from build123d import *

# Parameters (mm, degrees)
F0_W     = 23.8125
F0_H     = 7.9375
F0_R     = 2.38125
F1_DEPTH = 3.175
F2_DEPTH = 4.7625
F3_T     = -1.5875


with BuildPart() as f1:
    # F0 (on Top) → F1 (new body)
    with BuildSketch(Plane.XY):
        Rectangle(F0_W, F0_H)
        with Locations((-7.9375, 0)):
            Circle(F0_R, mode=Mode.SUBTRACT)
        Circle(F0_R, mode=Mode.SUBTRACT)
        with Locations((7.9375, 0)):
            Circle(F0_R, mode=Mode.SUBTRACT)
    extrude(amount=F1_DEPTH)

    # F0 (on Top) → F2 (join)
    with BuildSketch(Plane.XY):
        with Locations((-7.9375, 0)):
            Circle(F0_R)
        Circle(F0_R)
        with Locations((7.9375, 0)):
            Circle(F0_R)
    extrude(amount=F2_DEPTH)

    # F3
    f3_openings = [f1.faces().sort_by_distance(p)[0] for p in [
        (0, 0, 0),
    ]]
    offset(amount=F3_T, openings=f3_openings, kind=Kind.INTERSECTION)


solid = f1.part
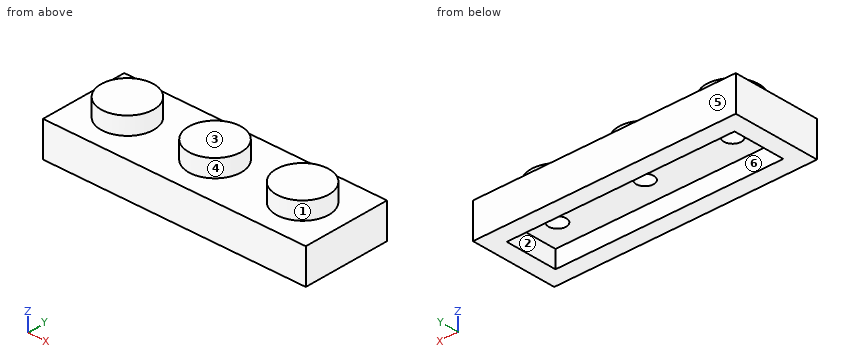
Design review of the part built by this model. Coordinates are the model's own, in mm. Face numbers are marked on the shaded views. A direction names the side the tool comes from. Give positions to 0.01 mm unless a question says otherwise; leave off trailing zeros. Loops run counter-clockwise (first coordinate to the right, second up) from the corner with the lowest first, then second, coordinate; pieces in that order, holes last. Notation, with made-up numbers: (-37.5, 53) -> (1.5, 53) arc R10 cw to (1.5, 65) -> close; hole circle Ø6 at (34.5, 41.25). An arc over 180 degrees is marked (long way). One line per question, with ' | ' between items. Start each with the question number.
(1) Draft analysis for pull direction Y (two halves, no side actions). For the marked faces 1, 2 and 3, state which applies: +Y half, -Y half, draft (parallel to the pull), parting line (faces both ways), or undercut.
(2) Insertion check: P1, Ø2.5, axis at x = 7.94, y = 0, coming from the -Z side; P2, Ø0.5, axis at x = 8, y = 0, coming from the -Z side (3 decimals). Each pin has a flat end and moves straight along its axis. Give the tip position at first contact, or say it passes through.
(3) We need section B-B (x = 0). State the section outline as (y, z) points (1 decimal).
(4) For line 1 (X direction, y = 0, z = 2.55); line 2 (X direction, y = 2.25, z = 0.35); line 3 (Y direction, x = -7, z = 0.5), list the stretches that pass through material, from the lowest coordinate up.
(5) We need section C-C (z = 1.95). State the section outline as (x, y) points, and give its area (3 significant figures).
(6) We need section A-A (z = 0.65). State the section outline as (x, y) points, and give its area (3 significant figures).
(7) For the marked faces 4, 5 and 6, list the 3-axis set-ups (+Z, -Z, +X, -X, +Y, -Y) from which the entire face can be reached by the end or side of a thin tool; tool diameter is ignored.
The answers:
1) face 1: parting line | face 2: undercut | face 3: draft
2) P1: stops at z = 1.59 | P2: stops at z = 3.175
3) outline: (-4, 0) -> (-2.4, 0) -> (-2.4, 1.6) -> (-0.8, 1.6) -> (-0.8, 3.2) -> (0.8, 3.2) -> (0.8, 1.6) -> (2.4, 1.6) -> (2.4, 0) -> (4, 0) -> (4, 3.2) -> (2.4, 3.2) -> (2.4, 4.8) -> (-2.4, 4.8) -> (-2.4, 3.2) -> (-4, 3.2) -> close
4) line 1: x = -11.91 to -8.73, -7.14 to -0.79, 0.79 to 7.14, 8.73 to 11.91 | line 2: x = -11.91 to -10.32, 10.32 to 11.91 | line 3: y = -3.97 to -2.38, 2.38 to 3.97
5) outline: (-11.91, -3.97) -> (11.91, -3.97) -> (11.91, 3.97) -> (-11.91, 3.97) -> close; hole circle Ø1.59 at (-7.94, 0); hole circle Ø1.59 at (0, 0); hole circle Ø1.59 at (7.94, 0) | area: 183 mm^2
6) outline: (-11.91, -3.97) -> (11.91, -3.97) -> (11.91, 3.97) -> (-11.91, 3.97) -> close; hole (-10.32, -2.38) -> (10.32, -2.38) -> (10.32, 2.38) -> (-10.32, 2.38) -> close | area: 90.7 mm^2
7) face 4: +Z | face 5: +Z, -Z, +X, -X, +Y | face 6: -Z
